```python
from build123d import *

# Parameters (mm, degrees)
SKETCH1_R               = 2.000000064
BOSS_EXTRUDE1_DEPTH     = 39.6875
SKETCH2_R               = 8.89
SKETCH2_R_2             = 6.35
CUT_EXTRUDE_THIN1_DEPTH = 7.9375


with BuildPart() as part:
    # Sketch1 → Boss-Extrude1 (new, symmetric)
    with BuildSketch(Plane.XY):
        Polygon((7.332348419, 0), (3.666174209, 6.35), (-3.666174209, 6.35), (-7.332348419, 0), (-3.666174209, -6.35), (3.666174209, -6.35), align=None)
        with Locations(Location((0, 0, 0), (0, 0, 180))):
            Circle(SKETCH1_R, mode=Mode.SUBTRACT)
    extrude(amount=BOSS_EXTRUDE1_DEPTH, both=True)

    # Sketch2 → Cut-Extrude-Thin1 (cut)
    with BuildSketch(Plane.XY.offset(31.75)):
        Circle(SKETCH2_R)
        Circle(SKETCH2_R_2, mode=Mode.SUBTRACT)
    cut_extrude_thin1 = extrude(amount=CUT_EXTRUDE_THIN1_DEPTH, mode=Mode.SUBTRACT)

    # Mirror1: Cut-Extrude-Thin1 across plane
    add(cut_extrude_thin1.mirror(Plane.XY), mode=Mode.SUBTRACT)


solid = part.part
```
Can you work these out from the model? Positions are in its coordinate system, mm. A direction names the side the tool comes from. Round coordinates to 2 decimals unless told otherwise and drop trailing zeros. Order: outer loops, then holes, each group sorted by start corner. A loop starts at its lowest first (then second) coordinate and runs counter-clockwise, first axis right, second up. Notation, with made-up numbers: (0.5, -15.75) -> (6.5, -15.75) arc R22 ccw to (6.5, 13.25) -> close; hole circle Ø11 at (41, 43). An arc over 180 degrees is marked (long way). Return JSON: item names as keys, results as strings. Group by question number.
1. If we section it at D-D, the plane y = 4.5: Write out the boundary of the cut face in (x, z), then the cut area to 4 significant figures.
2. If we section it at A-A, the plane z = 18: Write out the boundary of the cut face in (x, y).
3. Which directions (+Z, -Z, +X, -X, +Y, -Y) give clear straight access to the entire face, cutting with the end or side of a thin tool? Please do faces 1 (the face through (-1.38, -6.2, 35.66)), 2 (the face through (-3, 6, -31.75)), 3 (the face through (-1.38, -6.2, -35.66)).
4. If we section it at C-C, the plane x = 1: Write out the boundary of the cut face in (y, z), then the cut area to 3 significant figures.
5. Will these pins go through, and if not, where does the flat tip stop? pin 1 (0.5 mm diameter, centred on x = -6.5, y = -0.5, fed in from -Z); pin 2 (6 mm diameter, centred on y = -3.5, z = -20.5, fed in from -X); pin 3 (1.5 mm diameter, centred on y = -0.5, z = 8, fed in from -X).
6. We'd pull the mould along Y, two halves only. Please class faces 4 (the face through (-1.908, -0.601, -0.556)), 5 (the face through (-7, 0, -31.75)), 6 (the face through (5.474, -3.219, 0.445)): released by +Y, released by -Y, zero draft, split by the parting line, or undercut.
7. I need wall thicknesses on line 1 (X direction, y = 1.25, z = -35); line 2 (Z direction, x = -6, y = -2.25); line 3 (X direction, y = 1.25, z = 14). Which ranges of each line are inside material? Lowest first, please. Write a range as [from, to].
Output values:
{
 "1": {"outline": "(-4.73, -31.75) -> (-4.48, -31.75) -> (-4.48, -39.69) -> (4.48, -39.69) -> (4.48, -31.75) -> (4.73, -31.75) -> (4.73, 31.75) -> (4.48, 31.75) -> (4.48, 39.69) -> (-4.48, 39.69) -> (-4.48, 31.75) -> (-4.73, 31.75) -> close", "area": "743.5 mm²"},
 "2": {"outline": "(-7.33, 0) -> (-3.67, -6.35) -> (3.67, -6.35) -> (7.33, 0) -> (3.67, 6.35) -> (-3.67, 6.35) -> close; hole circle Ø4 at (0, 0)"},
 "3": {"face 1": "+Z", "face 2": "-Z, -X, +Y", "face 3": "-Z"},
 "4": {"outline": "(-6.35, -31.75) -> (-6.27, -31.75) -> (-6.27, -39.69) -> (-1.73, -39.69) -> (-1.73, 39.69) -> (-6.27, 39.69) -> (-6.27, 31.75) -> (-6.35, 31.75) -> close; (1.73, -39.69) -> (6.27, -39.69) -> (6.27, -31.75) -> (6.35, -31.75) -> (6.35, 31.75) -> (6.27, 31.75) -> (6.27, 39.69) -> (1.73, 39.69) -> close", "area": "731 mm²"},
 "5": {"pin 1": "z = -39.69", "pin 2": "x = -7.04", "pin 3": "x = -7.33"},
 "6": {"face 4": "undercut", "face 5": "zero draft", "face 6": "released by -Y"},
 "7": {"line 1": "[-6.23, -1.56], [1.56, 6.23]", "line 2": "[-31.75, 31.75]", "line 3": "[-6.61, -1.56], [1.56, 6.61]"}
}
